The model under review builds one solid part; all positions refer to its coordinate system, in mm. Face numbers are marked on the shaded views. A direction names the side the tool comes from. Coordinates: 2 decimals unless noted, no trailing zeros. Loops run counter-clockwise (first coordinate to the right, second up) from the corner with the lowest first, then second, coordinate; pieces in that order, holes last. Notation, with made-up numbers: (5, 11) - (43, 11) arc R26 ccw to (43, 39) - close; hole circle Ø6 at (89.25, 66.25). An arc over 180 degrees is marked (long way). Answer in a Markdown table with one row per item. Add a question column.
(1) We need section D-D on y = -44.5. Write out the cut boundary in (x, z), plus the area to 3 significant figures.
(2) We need section A-A on x = 0. Write out the cut boundary in (y, z).
(3) For line 1 along Y through (x, z) = (-35, -25); line 2 along X through (y, z) = (4, -40); line 3 along Z through (x, y) = (17, -35.5), list the stretches that pass through material, from the lowest coordinate up.
(4) We need section B-B on z = -40. Write out the cut boundary in (x, y), plus the area to 3 significant figures.
(5) We need section C-C on z = 21. Write out the cut boundary in (x, y), plus the area to 3 significant figures.
(6) Mouldability with a two-part tool opening along X and no side actions: class the marked faces 1, 2, 3 and 4 as +X half, -X half, draft (parallel to the pull), parting line (faces both ways), or undercut.
(7) Machinability: for the marked faces 5 and 6, which of the approach directions +Z, -Z, +X, -X, +Y, -Y give a long, thin tool a straight path to every point of the face, cutting with its end or side? Answer none if there is none.
(8) For P1, Ø4.5, axis at y = -37, z = 38.5, coming from the +X side; P2, Ø1.5, axis at x = -16, z = -34.5, coming from the +Y side; P3, Ø4.5, axis at y = -5.5, z = 24, coming from the +X side; P4, Ø4.5, axis at x = -35.5, y = -2, coming from the -Z side, all flat-tipped, find the tip position at first contact; note any pin that passes through.
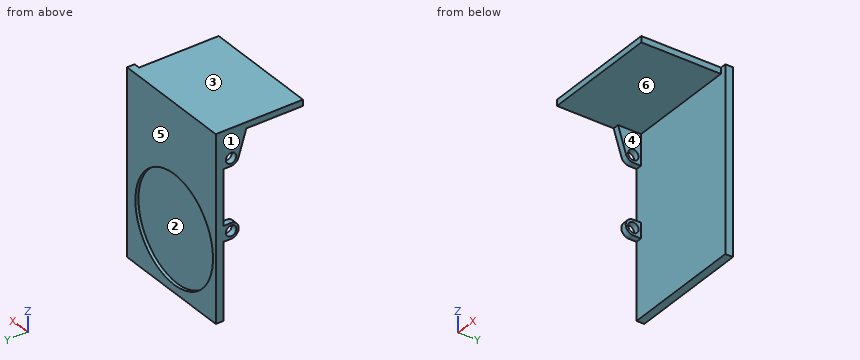
from build123d import *

# Parameters (mm, degrees)
SKETCH1_W           = 80
SKETCH1_H           = 120
BOSS_EXTRUDE1_DEPTH = 5
SKETCH2_W           = 76
SKETCH2_H           = 4
BOSS_EXTRUDE2_DEPTH = 52
SKETCH4_R           = 3.41
BOSS_EXTRUDE3_DEPTH = 4
SKETCH5_R           = 35
CUT_EXTRUDE1_DEPTH  = 2


with BuildPart() as part:
    # Sketch1 → Boss-Extrude1 (new body)
    with BuildSketch(Plane(origin=(0, 0, 0), x_dir=(1, 0, 0), z_dir=(0, 1, 0))):
        with Locations((2.5, 20)):
            Rectangle(SKETCH1_W, SKETCH1_H)
    extrude(amount=BOSS_EXTRUDE1_DEPTH)

    # Sketch2 → Boss-Extrude2 (add)
    with BuildSketch(Plane.XZ):
        with Locations((0.5, 38)):
            Rectangle(SKETCH2_W, SKETCH2_H)
    extrude(amount=BOSS_EXTRUDE2_DEPTH)

    # Sketch4 → Boss-Extrude3 (add)
    # profile 1 of 2: a face of its own
    with BuildSketch(Plane.ZY.offset(37.5)):
        with BuildLine():
            Line((-30, 0), (-20, 0))
            Line((-20, 0), (-20, -5))
            ThreePointArc((-20, -5), (-25, -10), (-30, -5))
            Line((-30, -5), (-30, 0))
        make_face()
        with Locations((-25, -5)):
            Circle(SKETCH4_R, mode=Mode.SUBTRACT)
    # profile 2 of 2: a face of its own
    with BuildSketch(Plane.ZY.offset(37.5)):
        with BuildLine():
            Line((16, 0), (16, -5))
            ThreePointArc((16, -5), (16.965508893, -7.953452473), (19.489152604, -9.766271094))
            Line((19.489152604, -9.766271094), (36, -15))
            Line((36, -15), (36, 0))
            Line((36, 0), (26, 0))
            Line((26, 0), (16, 0))
        make_face()
        with Locations(Location((21, -5, 0), (0, 0, 180))):
            Circle(SKETCH4_R, mode=Mode.SUBTRACT)
    extrude(amount=-BOSS_EXTRUDE3_DEPTH)

    # Sketch5 → Cut-Extrude1 (cut)
    with BuildSketch(Plane(origin=(0, 5, 0), x_dir=(1, 0, 0), z_dir=(0, 1, 0))):
        with Locations(Location((0, 40, 0), (0, 0, 270))):
            Circle(SKETCH5_R)
    extrude(amount=-CUT_EXTRUDE1_DEPTH, mode=Mode.SUBTRACT)


solid = part.part
Outcome:
| question | item | result |
|---|---|---|
| 1 | outline | (-37.5, 36) - (38.5, 36) - (38.5, 40) - (-37.5, 40) - close |
| 1 | area | 304 mm² |
| 2 | outline | (-52, 36) - (0, 36) - (0, -80) - (5, -80) - (5, -75) - (3, -75) - (3, -5) - (5, -5) - (5, 40) - (-52, 40) - close |
| 3 | line 1 | -10 to -8.41, -1.59 to 5 |
| 3 | line 2 | -37.5 to -35, 35 to 42.5 |
| 3 | line 3 | 36 to 40 |
| 4 | outline | (-37.5, 0) - (42.5, 0) - (42.5, 5) - (35, 5) - (35, 3) - (-35, 3) - (-35, 5) - (-37.5, 5) - close |
| 4 | area | 260 mm² |
| 5 | outline | (-37.5, -10.25) - (-33.5, -10.25) - (-33.5, -8.41) - (-37.5, -8.41) - close; (-37.5, -1.59) - (-33.5, -1.59) - (-33.5, 0) - (42.5, 0) - (42.5, 5) - (-37.5, 5) - close |
| 5 | area | 414 mm² |
| 6 | face 1 | -X half |
| 6 | face 2 | undercut |
| 6 | face 3 | draft |
| 6 | face 4 | +X half |
| 7 | face 5 | +Z, -Z, +X, -X, +Y |
| 7 | face 6 | -Z, +X, -Y |
| 8 | P1 | x = 38.5 |
| 8 | P2 | y = 3 |
| 8 | P3 | x = -33.5 |
| 8 | P4 | z = -80 |
